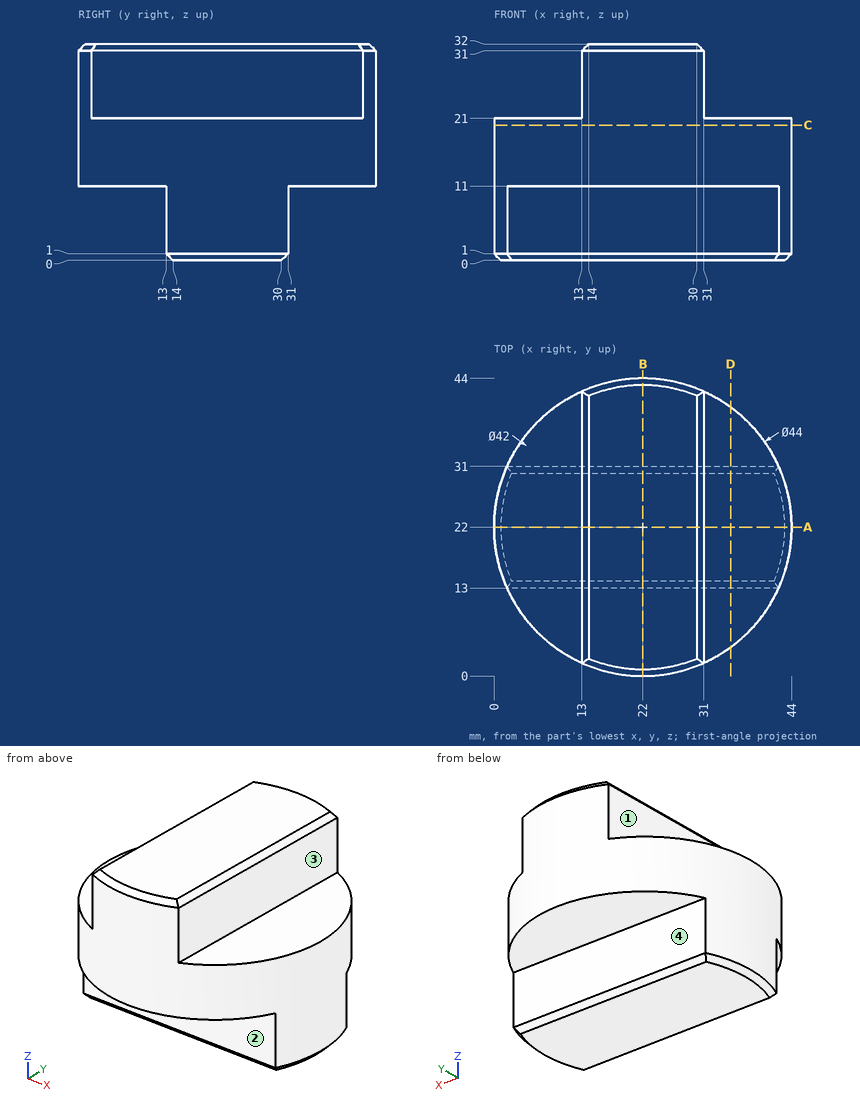
For this review, use the dimensioned drawing (mm, ordinates from the lowest corner) and the shaded views. A direction names the side the tool comes from. Coordinates: 2 decimals unless noted, no trailing zeros. Loops run counter-clockwise (first coordinate to the right, second up) from the corner with the lowest first, then second, coordinate; pieces in that order, holes last. Notation, with made-up numbers: (29, 68.25) -> (67, 68.25) arc R11 ccw to (67, 86.25) -> close; hole circle Ø8 at (24.5, 20). An arc over 180 degrees is marked (long way). Use a Markdown table: item, result. Add a question column.
1. Add section B-B on x = 22. Write out the cut boundary in (y, z).
2. To check wall thickness, follow line 1 (Y direction, x = 8.5, z = 8); line 2 (Z direction, x = 42, y = 21.5); line 3 (Z direction, x = 30, y = 8). State the ranges of each line that lie inside material, in increasing order.
3. Clearance check with flat-ended pins moving along their axes: pin 1 Ø8 at (y, z) = (21.5, 26.5) entering from -X; pin 2 Ø6.5 at (x, y) = (38.5, 23.5) entering from +Z; pin 3 Ø3 at (y, z) = (15, 25.5) entering from +X; pin 4 Ø14.5 at (x, y) = (7, 22.5) entering from +Z. State where each tip first meets the part, or that it passes through.
4. Add section C-C on z = 20. Write out the cut boundary in (x, y).
5. Add section A-A on y = 22. Write out the cut boundary in (x, z), plus the area to 3 significant figures.
6. Machinability: for the marked faces 1, 2, 3 and 4, which of the approach directions +Z, -Z, +X, -X, +Y, -Y give a long, thin tool a straight path to every point of the face, cutting with its end or side? Answer none if there is none.
7. Add section D-D on x = 35. Write out the cut boundary in (y, z).
Returned:
| question | item | result |
|---|---|---|
| 1 | outline | (0, 11) -> (13, 11) -> (13, 1) -> (14, 0) -> (30, 0) -> (31, 1) -> (31, 11) -> (44, 11) -> (44, 31) -> (43, 32) -> (1, 32) -> (0, 31) -> close |
| 2 | line 1 | y = 13 to 31 |
| 2 | line 2 | z = 0 to 21 |
| 2 | line 3 | z = 11 to 32 |
| 3 | pin 1 | stops at x = 13 |
| 3 | pin 2 | stops at z = 21 |
| 3 | pin 3 | stops at x = 31 |
| 3 | pin 4 | stops at z = 32 |
| 4 | outline | circle Ø44 at (22, 22) |
| 5 | outline | (0, 1) -> (1, 0) -> (43, 0) -> (44, 1) -> (44, 21) -> (31, 21) -> (31, 31) -> (30, 32) -> (14, 32) -> (13, 31) -> (13, 21) -> (0, 21) -> close |
| 5 | area | 1,120 mm² |
| 6 | face 1 | +Z, -X, +Y, -Y |
| 6 | face 2 | -Z, +X, -X, -Y |
| 6 | face 3 | +Z, +X, +Y, -Y |
| 6 | face 4 | -Z, +X, -X, +Y |
| 7 | outline | (4.25, 11) -> (13, 11) -> (13, 1) -> (14, 0) -> (30, 0) -> (31, 1) -> (31, 11) -> (39.75, 11) -> (39.75, 21) -> (4.25, 21) -> close |
